Work out the finished part from the listing and answer in its coordinate system (mm). Face numbers are marked on the shaded views. A direction names the side the tool comes from. Give positions to 0.01 mm unless a question says otherwise; leave off trailing zeros. Order: outer loops, then holes, each group sorted by start corner. A loop starts at its lowest first (then second) coordinate and runs counter-clockwise, first axis right, second up. Notation, with made-up numbers: (2, 35.5) - (36, 35.5) arc R20 ccw to (36, 64.5) - close; hole circle Ø9 at (-39, -23). An arc over 180 degrees is marked (long way). Put each result on its own line as item: value.
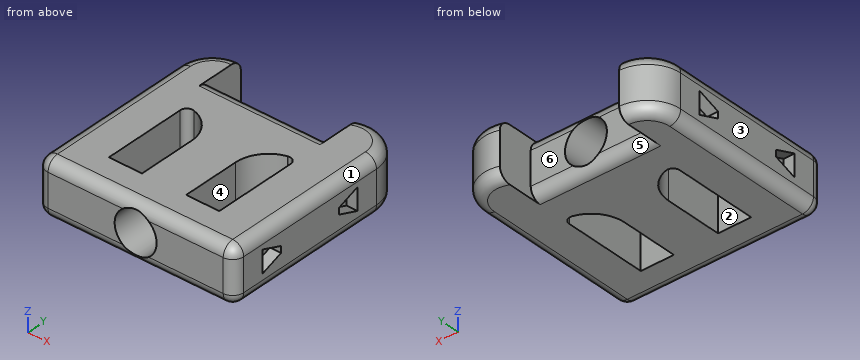
```python
from build123d import *

# Parameters (mm, degrees)
BOSS_EXTRUDE1_DEPTH = 25
SKETCH2_R           = 9.5
CUT_EXTRUDE1_DEPTH  = 89
FILLET1_R           = 5
FILLET2_R           = 5
FILLET3_R           = 5
CUT_EXTRUDE2_DEPTH  = 5


with BuildPart() as part:
    # Sketch1 → Boss-Extrude1 (new body)
    with BuildSketch(Plane.XY):
        with BuildLine():
            Line((83.342336402, -18.001464661), (83.342336402, -93))
            Line((83.342336402, -93), (-6, -93))
            Line((-6, -93), (-6, -18.001464661))
            ThreePointArc((-6, -18.001464661), (-1.606601718, -7.394862943), (9, -3.001464661))
            Line((9, -3.001464661), (9, -20))
            Line((9, -20), (63.671168201, -20))
            Line((63.671168201, -20), (63.671168201, -3.747335869))
            ThreePointArc((63.671168201, -3.747335869), (77.143827099, -5.855117), (83.342336402, -18.001464661))
        make_face()
        with BuildLine():
            Line((63.671168201, -40.39084965), (63.671168201, -78))
            Line((63.671168201, -78), (48.671168201, -78))
            Line((48.671168201, -78), (48.671168201, -52.009969466))
            ThreePointArc((48.671168201, -52.009969466), (51.788643958, -42.855428646), (59.845250549, -37.506095703))
            Line((59.845250549, -37.506095703), (59.905984671, -37.490074897))
            ThreePointArc((59.905984671, -37.490074897), (62.502076365, -38.014344801), (63.671168201, -40.39084965))
        make_face(mode=Mode.SUBTRACT)
        with BuildLine():
            Line((28.671168201, -78), (28.671168201, -52.009969466))
            ThreePointArc((28.671168201, -52.009969466), (25.553692444, -42.855428646), (17.497085853, -37.506095703))
            Line((17.497085853, -37.506095703), (17.436351731, -37.490074897))
            ThreePointArc((17.436351731, -37.490074897), (14.840260037, -38.014344801), (13.671168201, -40.39084965))
            Line((13.671168201, -40.39084965), (13.671168201, -78))
            Line((13.671168201, -78), (28.671168201, -78))
        make_face(mode=Mode.SUBTRACT)
    extrude(amount=BOSS_EXTRUDE1_DEPTH)

    # Sketch2 → Cut-Extrude1 (cut)
    with BuildSketch(Plane.XZ.offset(93)):
        with Locations(Location((38.671168201, 12.5, 0), (0, 0, 270))):
            Circle(SKETCH2_R)
    extrude(amount=-CUT_EXTRUDE1_DEPTH, mode=Mode.SUBTRACT)

    # Fillet1
    # the kernel refuses this fillet: 5 mm, written as the material it takes off along each edge
    with BuildSketch(Plane(origin=(95.842336402, -93, 0), x_dir=(0, 1, 0), z_dir=(-1, 0, 0))) as fillet1_piece_1:
        with BuildLine():
            CenterArc((FILLET1_R, -FILLET1_R), FILLET1_R, 90, 90)
            Line((0, -FILLET1_R), (0, 0))
            Line((0, 0), (FILLET1_R, 0))
        make_face()
    extrude(amount=114.342336402, mode=Mode.SUBTRACT)
    with BuildSketch(Plane(origin=(83.342336402, -93, -12.5), x_dir=(0, 1, 0), z_dir=(0, 0, 1)), Plane(origin=(-6, -93, -12.5), x_dir=(1, 0, 0), z_dir=(0, 0, 1))) as fillet1_piece_2:
        with BuildLine():
            CenterArc((FILLET1_R, FILLET1_R), FILLET1_R, 180, 90)
            Line((0, FILLET1_R), (0, 0))
            Line((0, 0), (FILLET1_R, 0))
        make_face()
    extrude(amount=50, mode=Mode.SUBTRACT)
    with BuildSketch(Plane(origin=(95.842336402, -93, 25), x_dir=(0, 1, 0), z_dir=(-1, 0, 0))) as fillet1_piece_3:
        with BuildLine():
            CenterArc((FILLET1_R, FILLET1_R), FILLET1_R, 180, 90)
            Line((0, FILLET1_R), (0, 0))
            Line((0, 0), (FILLET1_R, 0))
        make_face()
    extrude(amount=114.342336402, mode=Mode.SUBTRACT)

    # Fillet2
    # the kernel refuses this fillet: 5 mm, written as the material it takes off along each edge
    with BuildSketch(Plane(origin=(78.342336402, -88, 20), x_dir=(0, 0, 1), z_dir=(1, 0, 0))) as fillet2_piece_1_section:
        Polygon((0, 0), (FILLET2_R * 1.02, 0), (FILLET2_R * 1.02, FILLET2_R * 1.02), (0, FILLET2_R * 1.02), align=None)
    fillet2_piece_1 = extrude(amount=FILLET2_R * 1.02, mode=Mode.PRIVATE)
    fillet2_piece_1 = fillet2_piece_1 - Plane(origin=(78.342336402, -88, 20), x_dir=(0, 0.7071067811865475, -0.7071067811865475), z_dir=(1, 0, 0)) * Sphere(FILLET2_R, mode=Mode.PRIVATE)
    add(fillet2_piece_1, mode=Mode.SUBTRACT)
    with BuildSketch(Plane(origin=(78.342336402, -88, 5), x_dir=(0, 0, -1), z_dir=(1, 0, 0))) as fillet2_piece_2_section:
        Polygon((0, 0), (FILLET2_R * 1.02, 0), (FILLET2_R * 1.02, -FILLET2_R * 1.02), (0, -FILLET2_R * 1.02), align=None)
    fillet2_piece_2 = extrude(amount=FILLET2_R * 1.02, mode=Mode.PRIVATE)
    fillet2_piece_2 = fillet2_piece_2 - Plane(origin=(78.342336402, -88, 5), x_dir=(0, 0.7071067811865475, 0.7071067811865475), z_dir=(1, 0, 0)) * Sphere(FILLET2_R, mode=Mode.PRIVATE)
    add(fillet2_piece_2, mode=Mode.SUBTRACT)
    with BuildSketch(Plane(origin=(-1, -88, 20), x_dir=(-1, 0, 0), z_dir=(0, 0, 1))) as fillet2_piece_3_section:
        Polygon((0, 0), (FILLET2_R * 1.02, 0), (FILLET2_R * 1.02, FILLET2_R * 1.02), (0, FILLET2_R * 1.02), align=None)
    fillet2_piece_3 = extrude(amount=FILLET2_R * 1.02, mode=Mode.PRIVATE)
    fillet2_piece_3 = fillet2_piece_3 - Plane(origin=(-1, -88, 20), x_dir=(0.7071067811865476, 0.7071067811865475, 0), z_dir=(0, 0, 1)) * Sphere(FILLET2_R, mode=Mode.PRIVATE)
    add(fillet2_piece_3, mode=Mode.SUBTRACT)
    with BuildSketch(Plane(origin=(-1, -88, 5), x_dir=(-1, 0, 0), z_dir=(0, 0, -1))) as fillet2_piece_4_section:
        Polygon((0, 0), (FILLET2_R * 1.02, 0), (FILLET2_R * 1.02, -FILLET2_R * 1.02), (0, -FILLET2_R * 1.02), align=None)
    fillet2_piece_4 = extrude(amount=FILLET2_R * 1.02, mode=Mode.PRIVATE)
    fillet2_piece_4 = fillet2_piece_4 - Plane(origin=(-1, -88, 5), x_dir=(0.7071067811865476, 0.7071067811865475, 0), z_dir=(0, 0, -1)) * Sphere(FILLET2_R, mode=Mode.PRIVATE)
    add(fillet2_piece_4, mode=Mode.SUBTRACT)
    with BuildSketch(Plane(origin=(68.342336402, -18.001464661, 0), x_dir=(-0.9129658100806721, 0.4080360641214722, 0), z_dir=(-0.4080360641214722, -0.9129658100806721, 0))) as fillet2_piece_5_section:
        with BuildLine():
            CenterArc((15 - FILLET2_R, -FILLET2_R), FILLET2_R, 0, 90)
            Line((15 - FILLET2_R, 0), (15 - FILLET2_R, FILLET2_R * 0.02))
            Line((15 - FILLET2_R, FILLET2_R * 0.02), (15 + FILLET2_R * 0.02, FILLET2_R * 0.02))
            Line((15 + FILLET2_R * 0.02, FILLET2_R * 0.02), (15 + FILLET2_R * 0.02, -FILLET2_R))
            Line((15 + FILLET2_R * 0.02, -FILLET2_R), (15, -FILLET2_R))
        make_face()
    fillet2_piece_5 = revolve(axis=Axis((68.342336402, -18.001464661, 0), (0, 0, -1)), revolution_arc=155.918477011, mode=Mode.PRIVATE)
    fillet2_piece_5 = split(fillet2_piece_5, bisect_by=Plane(origin=(63.671168201, -6.375046545, 1.425351683), z_dir=(1, 0, 0)), keep=Keep.TOP, mode=Mode.PRIVATE)
    add(fillet2_piece_5, mode=Mode.SUBTRACT)
    with BuildSketch(Plane(origin=(-6, -88, 0), x_dir=(1, 0, 0), z_dir=(0, 1, 0)), Plane(origin=(83.342336402, -18.001464661, 25), x_dir=(0, 0, -1), z_dir=(0, -1, 0))) as fillet2_piece_6:
        with BuildLine():
            CenterArc((FILLET2_R, -FILLET2_R), FILLET2_R, 90, 90)
            Line((0, -FILLET2_R), (-FILLET2_R * 0.02, -FILLET2_R))
            Line((-FILLET2_R * 0.02, -FILLET2_R), (-FILLET2_R * 0.02, FILLET2_R * 0.02))
            Line((-FILLET2_R * 0.02, FILLET2_R * 0.02), (FILLET2_R, FILLET2_R * 0.02))
            Line((FILLET2_R, FILLET2_R * 0.02), (FILLET2_R, 0))
        make_face()
    extrude(amount=69.998535339, mode=Mode.SUBTRACT)
    with BuildSketch(Plane(origin=(68.342336402, -18.001464661, 25), x_dir=(-0.9129658100806721, 0.4080360641214721, 0), z_dir=(-0.4080360641214721, -0.9129658100806721, 0))) as fillet2_piece_7_section:
        with BuildLine():
            CenterArc((15 - FILLET2_R, FILLET2_R), FILLET2_R, 270, 90)
            Line((15 - FILLET2_R, 0), (15 - FILLET2_R, -FILLET2_R * 0.02))
            Line((15 - FILLET2_R, -FILLET2_R * 0.02), (15 + FILLET2_R * 0.02, -FILLET2_R * 0.02))
            Line((15 + FILLET2_R * 0.02, -FILLET2_R * 0.02), (15 + FILLET2_R * 0.02, FILLET2_R))
            Line((15 + FILLET2_R * 0.02, FILLET2_R), (15, FILLET2_R))
        make_face()
    fillet2_piece_7 = revolve(axis=Axis((68.342336402, -18.001464661, 25), (0, 0, -1)), revolution_arc=155.918477011, mode=Mode.PRIVATE)
    fillet2_piece_7 = split(fillet2_piece_7, bisect_by=Plane(origin=(63.671168201, -6.375046545, 23.574648317), z_dir=(1, 0, 0)), keep=Keep.TOP, mode=Mode.PRIVATE)
    add(fillet2_piece_7, mode=Mode.SUBTRACT)
    with BuildSketch(Plane(origin=(9, -18.001464661, 25), x_dir=(-1, 0, 0), z_dir=(0, -1, 0))) as fillet2_piece_8:
        with BuildLine():
            CenterArc((15 - FILLET2_R, FILLET2_R), FILLET2_R, 270, 90)
            Line((15, FILLET2_R), (15 + FILLET2_R * 0.02, FILLET2_R))
            Line((15 + FILLET2_R * 0.02, FILLET2_R), (15 + FILLET2_R * 0.02, -FILLET2_R * 0.02))
            Line((15 + FILLET2_R * 0.02, -FILLET2_R * 0.02), (15 - FILLET2_R, -FILLET2_R * 0.02))
            Line((15 - FILLET2_R, -FILLET2_R * 0.02), (15 - FILLET2_R, 0))
        make_face()
    revolve(axis=Axis((9, -18.001464661, 25), (0, 0, -1)), revolution_arc=90, mode=Mode.SUBTRACT)
    with BuildSketch(Plane(origin=(-6, -88, 25), x_dir=(1, 0, 0), z_dir=(0, 1, 0)), Plane(origin=(83.342336402, -18.001464661, 0), x_dir=(0, 0, 1), z_dir=(0, -1, 0))) as fillet2_piece_9:
        with BuildLine():
            CenterArc((FILLET2_R, FILLET2_R), FILLET2_R, 180, 90)
            Line((0, FILLET2_R), (-FILLET2_R * 0.02, FILLET2_R))
            Line((-FILLET2_R * 0.02, FILLET2_R), (-FILLET2_R * 0.02, -FILLET2_R * 0.02))
            Line((-FILLET2_R * 0.02, -FILLET2_R * 0.02), (FILLET2_R, -FILLET2_R * 0.02))
            Line((FILLET2_R, -FILLET2_R * 0.02), (FILLET2_R, 0))
        make_face()
    extrude(amount=69.998535339, mode=Mode.SUBTRACT)
    with BuildSketch(Plane(origin=(9, -18.001464661, 0), x_dir=(-1, 0, 0), z_dir=(0, -1, 0))) as fillet2_piece_10:
        with BuildLine():
            CenterArc((15 - FILLET2_R, -FILLET2_R), FILLET2_R, 0, 90)
            Line((15, -FILLET2_R), (15 + FILLET2_R * 0.02, -FILLET2_R))
            Line((15 + FILLET2_R * 0.02, -FILLET2_R), (15 + FILLET2_R * 0.02, FILLET2_R * 0.02))
            Line((15 + FILLET2_R * 0.02, FILLET2_R * 0.02), (15 - FILLET2_R, FILLET2_R * 0.02))
            Line((15 - FILLET2_R, FILLET2_R * 0.02), (15 - FILLET2_R, 0))
        make_face()
    revolve(axis=Axis((9, -18.001464661, 0), (0, 0, -1)), revolution_arc=90, mode=Mode.SUBTRACT)

    # Fillet3
    # the kernel refuses this fillet: 5 mm, written as the material it takes off along each edge
    with BuildSketch(Plane(origin=(9, -20, 25), x_dir=(0, -1, 0), z_dir=(1, 0, 0))) as fillet3_piece_1:
        with BuildLine():
            CenterArc((FILLET3_R, FILLET3_R), FILLET3_R, 180, 90)
            Line((0, FILLET3_R), (0, 0))
            Line((0, 0), (FILLET3_R, 0))
        make_face()
    extrude(amount=54.671168201, mode=Mode.SUBTRACT)
    with BuildSketch(Plane(origin=(9, -20, 0), x_dir=(0, -1, 0), z_dir=(1, 0, 0))) as fillet3_piece_2:
        with BuildLine():
            CenterArc((FILLET3_R, -FILLET3_R), FILLET3_R, 90, 90)
            Line((0, -FILLET3_R), (0, 0))
            Line((0, 0), (FILLET3_R, 0))
        make_face()
    extrude(amount=54.671168201, mode=Mode.SUBTRACT)

    # Sketch3 → Cut-Extrude2 (cut)
    with BuildSketch(Plane(origin=(83.342336402, 0, 0), x_dir=(0, 0, -1), z_dir=(1, 0, 0))):
        Polygon((-17.768000409, -28.001464661), (-7.768000409, -28.001464661), (-11.294178767, -37.689560075), (-14.241822052, -37.689560075), align=None)
        Polygon((-11.294178767, -68.311904586), (-14.241822052, -68.311904586), (-17.768000409, -78), (-7.768000409, -78), align=None)
    cut_extrude2 = extrude(amount=-CUT_EXTRUDE2_DEPTH, mode=Mode.SUBTRACT)

    # Mirror1: Cut-Extrude2 across plane
    add(cut_extrude2.mirror(Plane(origin=(38.671168201, 0, 0), x_dir=(0, 0, 1), z_dir=(1, 0, 0))), mode=Mode.SUBTRACT)


solid = part.part
```
(1) Given pin 1 (4.5 mm diameter, centred on x = 18.5, z = 9.5, fed in from +Y); pin 2 (1.5 mm diameter, centred on x = 80, z = 13, fed in from +Y); pin 3 (3 mm diameter, centred on y = -32.5, z = 13.5, fed in from -X), each flat-ended and moving along its own axis, determine where each tip first touches the part or whether it passes through.
Geometry check:
pin 1: stops at y = -20
pin 2: stops at y = -7.7
pin 3: stops at x = -1
(2) Section C-C, the plane x = 50 is taken. Write down the section's boundary in (y, z), then the cut area to 3 significant figures.
Geometry check:
outline: (-93, 5) arc R5 ccw to (-88, 0) - (-78, 0) - (-78, 25) - (-88, 25) arc R5 ccw to (-93, 20) - close; (-45.84, 0) - (-25, 0) arc R5 ccw to (-20, 5) - (-20, 20) arc R5 ccw to (-25, 25) - (-45.84, 25) - close
area: 999 mm²
(3) Determine the mould class of the marked faces 1, 2 and 3 for opening direction X: pulls with the +X half, pulls with the -X half, needs draft (parallel to the pull), parting line crosses it, or undercut.
Geometry check:
face 1: pulls with the +X half
face 2: undercut
face 3: pulls with the -X half
(4) Section D-D, the plane y = -29.5 is taken. Write down the section's boundary in (x, z).
Geometry check:
outline: (-6, 5) arc R5 ccw to (-1, 0) - (78.34, 0) arc R5 ccw to (83.34, 5) - (83.34, 8.31) - (78.34, 8.31) - (78.34, 17.22) - (83.34, 17.22) - (83.34, 20) arc R5 ccw to (78.34, 25) - (-1, 25) arc R5 ccw to (-6, 20) - (-6, 17.22) - (-1, 17.22) - (-1, 8.31) - (-6, 8.31) - close; hole circle Ø19 at (38.67, 12.5)
(5) Straight lines are drawn through the part: line 1 (X direction, y = -72, z = 12.5); line 2 (X direction, y = -55.5, z = 12.5); line 3 (Y direction, x = 16.5, z = 19.25). For each, find the intervals that lie inside material, in ascending order.
Geometry check:
line 1: x = -1 to 13.67, 28.67 to 29.17, 48.17 to 48.67, 63.67 to 78.34
line 2: x = -6 to 13.67, 28.67 to 29.17, 48.17 to 48.67, 63.67 to 83.34
line 3: y = -93 to -78, -37.4 to -20
(6) Section A-A, the plane y = -43 is taken. Write down the section's boundary in (x, z), then the cut area to 3 significant figures.
Geometry check:
outline: (-6, 5) arc R5 ccw to (-1, 0) - (13.67, 0) - (13.67, 25) - (-1, 25) arc R5 ccw to (-6, 20) - close; (25.66, 0) - (51.68, 0) - (51.68, 25) - (25.66, 25) - close; (63.67, 0) - (78.34, 0) arc R5 ccw to (83.34, 5) - (83.34, 20) arc R5 ccw to (78.34, 25) - (63.67, 25) - close; hole circle Ø19 at (38.67, 12.5)
area: 1,330 mm²
(7) A tool of negligible diameter and unlimited length cuts with its end or side. For the marked faces 4, 5 and 6, from which of +Z, -Z, +X, -X, +Y, -Y can it reach the whole face along a straight path? Write none if from no direction.
Geometry check:
face 4: +Z, -Z
face 5: -Z, +Y
face 6: +Z, -Z, +Y
(8) Section B-B, the plane z = 12.5 is taken. Count the separate pieces of the cut face and the enclosed holes in it, then the cut area to 3 significant figures.
Geometry check:
separate pieces: 2
enclosed holes: 2
area: 4,290 mm²
